Study the drawing (mm; zero at the part's minimum x, y, z) and answer. A direction names the side the tool comes from. Coordinates: 2 decimals unless noted, no trailing zeros. Write each loop counter-clockwise with the first axis right and the second up, starting at its lowest first coordinate (ties: lowest second). Pieces come first, ordered by that corner, then holes. Notation, with made-up numbers: (50.25, -14.75) -> (61.25, -14.75) arc R30 cw to (61.25, 19.25) -> close; hole circle Ø11 at (17.5, 48.25). An arc over 180 degrees is marked (long way). Answer in a Markdown table with one row per item. Add a question column.
Item 1: Straight lines are drawn through the part: line 1 (Z direction, x = 5.75, y = 10.5); line 2 (X direction, y = 10.5, z = 5) (1 decimal); line 3 (X direction, y = 14, z = 4) (1 decimal). For each, find the intervals that lie inside material, in ascending order. Write a range as from..to.
Item 2: Section C-C on x = 6 is taken. Write down the section's boundary in (y, z).
Item 3: Given pin 1 Ø2 at (x, y) = (5, 12) entering from +Z; pin 2 Ø3 at (y, z) = (17.5, 4.5) entering from +X (1 decimal); pin 3 Ø4 at (y, z) = (2.5, 1) entering from -X, each flat-ended and moving along its own axis, determine where each tip first touches the part or whether it passes through.
Item 4: Which of the six approach directions +Z, -Z, +X, -X, +Y, -Y give full straight-line access (tool end or side, diameter ignored) to the marked faces 1 and 2?
Item 5: Section D-D on x = 7.75 is taken. Write down the section's boundary in (y, z).
Item 6: Section B-B on z = 5.5 is taken. Write down the section's boundary in (x, y).
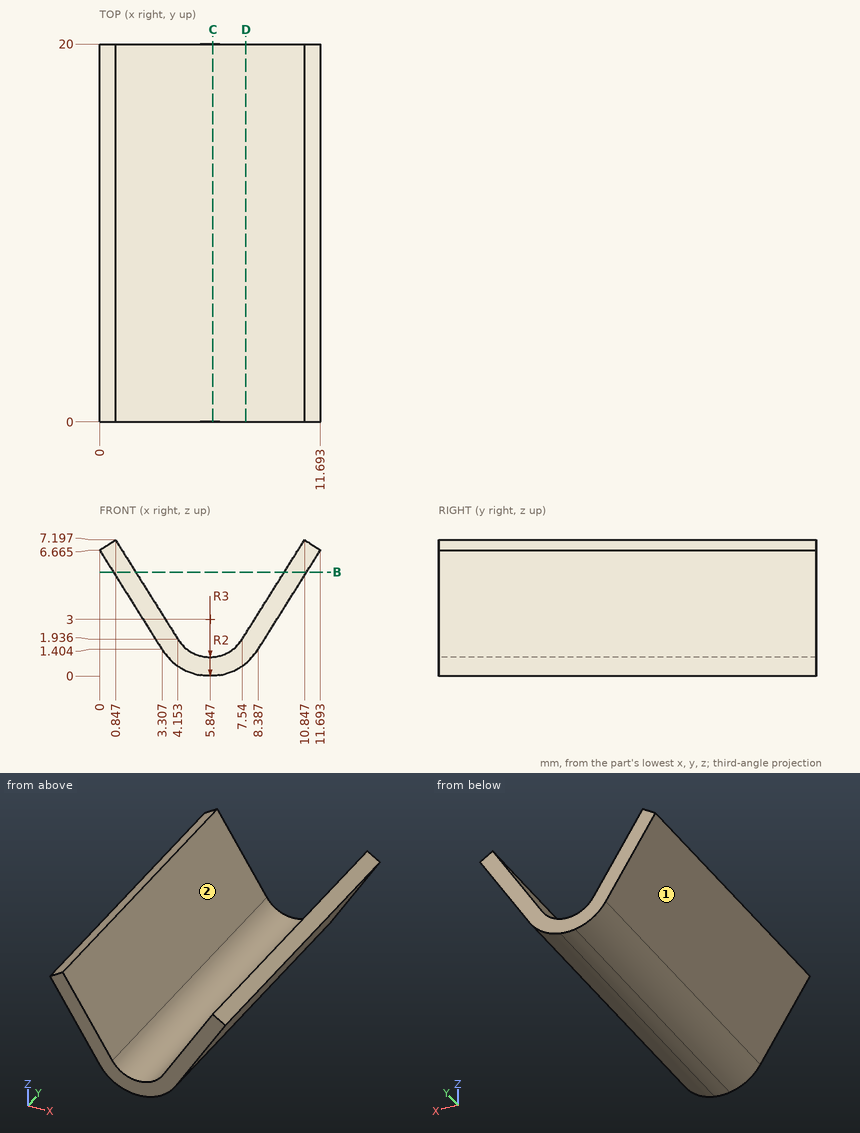
Results below:
| question | item | result |
|---|---|---|
| 1 | line 1 | z = 0..1 |
| 1 | line 2 | x = 1..2.2, 9.5..10.6 |
| 1 | line 3 | x = 1.7..2.9, 8.8..10 |
| 2 | outline | (0, 0) -> (20, 0) -> (20, 1.01) -> (0, 1.01) -> close |
| 3 | pin 1 | stops at z = 2.18 |
| 3 | pin 2 | stops at x = 11.3 |
| 3 | pin 3 | stops at x = 2.3 |
| 4 | face 1 | -Z, -X, +Y, -Y |
| 4 | face 2 | +Z, +Y, -Y |
| 5 | outline | (0, 0.68) -> (20, 0.68) -> (20, 2.27) -> (0, 2.27) -> close |
| 6 | outline | (0.73, 0) -> (1.91, 0) -> (1.91, 20) -> (0.73, 20) -> close; (9.78, 0) -> (10.96, 0) -> (10.96, 20) -> (9.78, 20) -> close |
